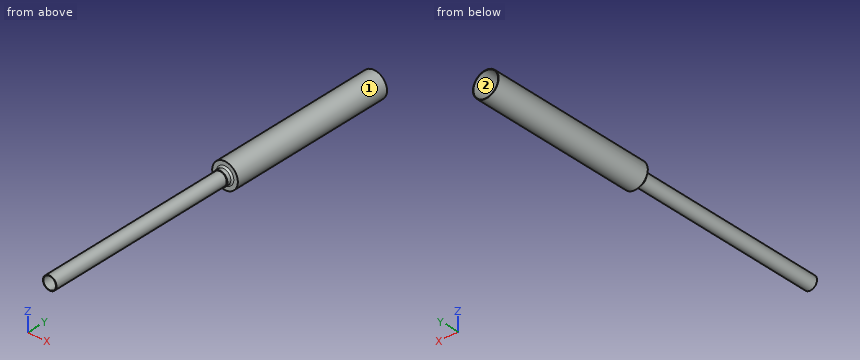
Autodesk Inventor part; units mm, degrees
ref_plane "YZ Plane" through (0, 0, 0) normal (1, 0, 0) x (0, 1, 0)
ref_plane "XZ Plane" through (0, 0, 0) normal (0, 1, 0) x (-1, 0, 0)
ref_plane "XY Plane" through (0, 0, 0) normal (0, 0, 1) x (1, 0, 0)
sketch "Sketch1" plane through (0, 0, 0) normal (0, 1, 0) x (-1, 0, 0)
  circle A0 centre (0, 0) radius 25.4635
  circle A1 centre (0, 0) radius 24.5237
  dimension "d0" = 50.927
  dimension "d1" = 0.9398
extrude "Extrusion1" add sketch "Sketch1" against normal blind 332.5
sketch "Sketch2" plane through (0, -332.5, 0) normal (0, -1, 0) x (1, 0, 0)
  circle A0 centre (0, 0) radius 14.2875
  circle A1 centre (0, 0) radius 25.4635
  circle A2 centre (0, 0) radius 25.4635
  dimension "d4" = 28.575
extrude "Extrusion2" add sketch "Sketch2" along normal blind 0.9398
sketch "Sketch3" plane through (0, -332.5, 0) normal (0, 1, 0) x (1, 0, 0)
  circle A0 centre (0, 0) radius 14.2875
  circle A1 centre (0, 0) radius 14.2875
  circle A2 centre (0, 0) radius 13.3477
  dimension "d7" = 0.9398
extrude "Extrusion3" add sketch "Sketch3" against normal blind 11.811
sketch "Sketch4" plane through (0, -344.311, 0) normal (0, -1, 0) x (1, 0, 0)
  circle A0 centre (0, 0) radius 13.3477
  circle A1 centre (0, 0) radius 13.3477
  circle A2 centre (0, 0) radius 12.4079
  dimension "d10" = 0.9398
extrude "Extrusion4" add sketch "Sketch4" along normal blind 381 and the other way blind 5.08
fillet "Fillet1" radius 3.175 1 edges at (-14.2875, -333.4398, 0)
fillet "Fillet2" radius 0.508 1 edges at (-13.3477, -344.311, 0)
properties part number "still pipe unmodified" material "Stainless Steel AISI 304"
Source: CAD feature listing. Evaluate the final solid. Frame: model axes, mm. Face numbers are marked on the shaded views. Coordinates: 2 decimals unless noted, no trailing zeros. Write each loop counter-clockwise with the first axis right and the second up, starting at its lowest first coordinate (ties: lowest second). Pieces come first, ordered by that corner, then holes. Notation, with made-up numbers: (22.5, 41.25) -> (67.5, 41.25) arc R21 cw to (67.5, 67.25) -> close; hole circle Ø6 at (74, 9.25). An arc over 180 degrees is marked (long way). Return JSON: item names as keys, results as strings. Group by question number.
1) Section query C-C, the plane y = -420. Return loops of the section in (x, z).
2) Mould query, pull axis Z, two halves, no side actions, for the marked faces 1 and 2. Classes: +Z half, -Z half, draft (parallel to the pull), parting line (faces both ways), or undercut.
3) Section query D-D, the plane y = -125. Return loops of the section in (x, z), plus the area to 3 significant figures.
4) Contact query for flat-ended pins moving along their axis: P1, Ø2, axis at x = 12, z = -6, coming from the -Y side; P2, Ø1.5, axis at x = -6.5, y = -446, coming from the +Z side; P3, Ø4, axis at y = -296.5, z = 8, coming from the +X side; P4, Ø1.5, axis at y = -362, z = 5.5, coming from the +X side. Output: stop coordinate, or through.
5) Ray query, line 1 along X through (y, z) = (-337, 0); line 2 along Z through (x, y) = (-2.5, -316.5); line 3 along Z through (x, y) = (0, -336). Return the intervals inside material, ascending.
From the geometry:
{
 "1": {"outline": "circle Ø26.7 at (0, 0); hole circle Ø24.82 at (0, 0)"},
 "2": {"face 1": "parting line", "face 2": "undercut"},
 "3": {"outline": "circle Ø50.93 at (0, 0); hole circle Ø49.05 at (0, 0)", "area": "148 mm²"},
 "4": {"P1": "y = -725.31", "P2": "z = 12.05", "P3": "x = 24.75", "P4": "x = 12.47"},
 "5": {"line 1": "-14.29 to -13.35, 13.35 to 14.29", "line 2": "-25.34 to -24.4, 24.4 to 25.34", "line 3": "-14.35 to -13.35, 13.35 to 14.35"}
}
